from build123d import *

# Parameters (mm, degrees)
CROQUIS1_R              = 32
CROQUIS1_R_2            = 1.7
SALIENTE_EXTRUIR1_DEPTH = 2.5
CROQUIS2_R              = 16
CROQUIS2_R_2            = 11
SALIENTE_EXTRUIR2_DEPTH = 7
CROQUIS3_R              = 5
CORTAR_EXTRUIR1_DEPTH   = 7


with BuildPart() as part:
    # Croquis1 → Saliente-Extruir1 (new body)
    with BuildSketch(Plane(origin=(0, 0, 0), x_dir=(1, 0, 0), z_dir=(0, 1, 0))):
        with Locations(Location((0, 0, 0), (0, 0, 270))):
            Circle(CROQUIS1_R)
        with Locations(Location((29, 0, 0), (0, 0, 270))):
            Circle(CROQUIS1_R_2, mode=Mode.SUBTRACT)
        with Locations(Location((-29, 0, 0), (0, 0, 270))):
            Circle(CROQUIS1_R_2, mode=Mode.SUBTRACT)
        with Locations(Location((0, 29, 0), (0, 0, 270))):
            Circle(CROQUIS1_R_2, mode=Mode.SUBTRACT)
    extrude(amount=SALIENTE_EXTRUIR1_DEPTH)

    # Croquis2 → Saliente-Extruir2 (add)
    with BuildSketch(Plane.XZ):
        with Locations(Location((0, 0, 0), (0, 0, 90))):
            Circle(CROQUIS2_R)
        with Locations(Location((0, 0, 0), (0, 0, 270))):
            Circle(CROQUIS2_R_2, mode=Mode.SUBTRACT)
    extrude(amount=SALIENTE_EXTRUIR2_DEPTH)

    # Croquis3 → Cortar-Extruir1 (cut)
    with BuildSketch(Plane.XZ):
        with Locations(Location((0, 0, 0), (0, 0, 270))):
            Circle(CROQUIS3_R)
    extrude(amount=-CORTAR_EXTRUIR1_DEPTH, mode=Mode.SUBTRACT)


solid = part.part
Input: part model. Units: mm. Frame: model coordinates. A direction names the side the tool comes from. Coordinates: 2 decimals unless noted, no trailing zeros. Loops run counter-clockwise (first coordinate to the right, second up) from the corner with the lowest first, then second, coordinate; pieces in that order, holes last. Notation, with made-up numbers: (29.25, 87.25) - (42.25, 87.25) arc R25 ccw to (42.25, 123.25) - close; hole circle Ø9 at (78.25, 71.25). An arc over 180 degrees is marked (long way). Answer in a Markdown table with one row per item. Add a question column.
Item 1: Access query for faces 4 (the flat face through (15, 0, 7)), 5 (the flat face through (0, 2.5, 7)). Directions: +Z, -Z, +X, -X, +Y, -Y. A direction counts if a zero-diameter tool reaches every point of the face in a straight line with its end or side. Return the directions, or none.
Item 2: Section query A-A on x = 0. Return the cut outline in (y, z), then the cut area to 4 significant figures.
Item 3: Contact query for flat-ended pins moving along their axis: P1, Ø2, axis at y = -5.5, z = 7.5, coming from the +X side; P2, Ø24, axis at x = -4, z = 2, coming from the -Y side; P3, Ø5, axis at x = 0.5, y = -5.5, coming from the +Z side; P4, Ø4.5, axis at x = 29, z = 0, coming from the -Y side. Output: stop coordinate, or through.
Item 4: Section query B-B on z = 0. Return the cut outline in (x, y).
Item 5: Section query D-D on y = -5.5. Return the cut outline in (x, z).
Item 6: Line query: line 1 along X through (y, z) = (1.25, 0); line 2 along Y through (x, z) = (-18.5, -26); line 3 along X through (y, z) = (-4.5, 0). Output: solid intervals per line, ascending. Write a range as [from, to].
Item 7: Mould query, pull axis X, two halves, no side actions, for faces 1 (the cylindrical face through (-31.24, 1.23, -6.94)), 2 (the flat face through (-11, -7, 3)), 3 (the cylindrical face through (-10.74, -3.45, 2.38)). Classes: released by +X, released by -X, zero draft, split by the parting line, or undercut.
Item 8: Section query C-C on x = 29. Return the cut outline in (y, z).
Recorded:
| question | item | result |
|---|---|---|
| 1 | face 4 | -Y |
| 1 | face 5 | +Z, -Z, +X, -X, +Y |
| 2 | outline | (-7, -16) - (0, -16) - (0, -27.3) - (2.5, -27.3) - (2.5, -5) - (0, -5) - (0, -11) - (-7, -11) - close; (-7, 11) - (0, 11) - (0, 5) - (2.5, 5) - (2.5, 32) - (0, 32) - (0, 16) - (-7, 16) - close; (0, -32) - (2.5, -32) - (2.5, -30.7) - (0, -30.7) - close |
| 2 | area | 196.5 mm^2 |
| 3 | P1 | x = 14.62 |
| 3 | P2 | y = -7 |
| 3 | P3 | z = 16 |
| 3 | P4 | y = 0 |
| 4 | outline | (-32, 0) - (-30.7, 0) - (-30.7, 2.5) - (-32, 2.5) - close; (-27.3, 0) - (-16, 0) - (-16, -7) - (-11, -7) - (-11, 0) - (-5, 0) - (-5, 2.5) - (-27.3, 2.5) - close; (5, 0) - (11, 0) - (11, -7) - (16, -7) - (16, 0) - (27.3, 0) - (27.3, 2.5) - (5, 2.5) - close; (30.7, 0) - (32, 0) - (32, 2.5) - (30.7, 2.5) - close |
| 5 | outline | circle Ø32 at (0, 0); hole circle Ø22 at (0, 0) |
| 6 | line 1 | [-32, -30.7], [-27.3, -5], [5, 27.3], [30.7, 32] |
| 6 | line 2 | [0, 2.5] |
| 6 | line 3 | [-16, -11], [11, 16] |
| 7 | face 1 | split by the parting line |
| 7 | face 2 | zero draft |
| 7 | face 3 | undercut |
| 8 | outline | (0, -13.53) - (2.5, -13.53) - (2.5, -1.7) - (0, -1.7) - close; (0, 1.7) - (2.5, 1.7) - (2.5, 13.53) - (0, 13.53) - close |
